from build123d import *

# Parameters (mm, degrees)
SKETCH1_W                                       = 22
SKETCH1_H                                       = 22
BOSS_EXTRUDE1_DEPTH                             = 10
F_1_4_CLEARANCE_HOLE1_D                         = 6.7564
SKETCH6_R                                       = 4
CUT_EXTRUDE1_DEPTH                              = 207.717198123
SKETCH7_R                                       = 12
CUT_EXTRUDE2_DEPTH                              = 207.717198123
CBORE_FOR_10_SOCKET_HEAD_CAP_SCREW1_D           = 5.6134
CBORE_FOR_10_SOCKET_HEAD_CAP_SCREW1_CBORE_D     = 9.525
CBORE_FOR_10_SOCKET_HEAD_CAP_SCREW1_CBORE_DEPTH = 4.826
BOSS_EXTRUDE2_DEPTH                             = 10
BOSS_EXTRUDE2_DEPTH_BACK                        = 10
CBORE_FOR_M3_SHCS1_D                            = 3.6
CBORE_FOR_M3_SHCS1_CBORE_D                      = 6.5
CBORE_FOR_M3_SHCS1_CBORE_DEPTH                  = 3
FILLET1_R                                       = 3
FILLET2_R                                       = 3
FILLET3_R                                       = 10
FILLET4_R                                       = 2


with BuildPart() as part:
    # Sketch1 → Boss-Extrude1 (new body)
    with BuildSketch(Plane(origin=(0, 0, 0), x_dir=(1, 0, 0), z_dir=(0, 1, 0))):
        with Locations((15, 15)):
            Rectangle(SKETCH1_W, SKETCH1_H)
        Polygon((50, 50), (50, 58.485281374), (17.514718626, 26), (26, 26), (26, 17.514718626), (58.485281374, 50), align=None)
        Polygon((50, 75), (50, 100), (75, 100), (100, 100), (100, 50), (75, 50), (50, 50), align=None)
        Polygon((100, 50), (91.514718626, 50), (124, 17.514718626), (124, 26), (132.485281374, 26), (100, 58.485281374), align=None)
        with Locations((135, 15)):
            Rectangle(SKETCH1_W, SKETCH1_H)
        with Locations((135, 135)):
            Rectangle(SKETCH1_W, SKETCH1_H)
        Polygon((124, 132.485281374), (91.514718626, 100), (100, 100), (100, 91.514718626), (132.485281374, 124), (124, 124), align=None)
        Polygon((17.514718626, 124), (50, 91.514718626), (50, 100), (58.485281374, 100), (26, 132.485281374), (26, 124), align=None)
        with Locations((15, 135)):
            Rectangle(SKETCH1_W, SKETCH1_H)
    extrude(amount=-BOSS_EXTRUDE1_DEPTH)

    # 1/4 Clearance Hole1 (through all)
    with Locations(Plane(origin=(0, 0, 0), x_dir=(1, 0, 0), z_dir=(0, 1, 0))):
        with Locations((15, 15), (15, 135), (135, 135), (135, 15)):
            Hole(F_1_4_CLEARANCE_HOLE1_D / 2)

    # Sketch6 → Cut-Extrude1 (cut, through all)
    with BuildSketch(Plane.XZ.offset(10)):
        with Locations(Location((75, -75, 0), (0, 0, 270))):
            Circle(SKETCH6_R)
    extrude(amount=-CUT_EXTRUDE1_DEPTH, mode=Mode.SUBTRACT)

    # Sketch7 → Cut-Extrude2 (cut, through all)
    with BuildSketch(Plane(origin=(0, -10, 0), x_dir=(1, 0, 0), z_dir=(0, 1, 0))):
        with Locations(Location((75, 75, 0), (0, 0, 270))):
            Circle(SKETCH7_R)
    extrude(amount=CUT_EXTRUDE2_DEPTH, mode=Mode.SUBTRACT)

    # CBORE for #10 Socket Head Cap Screw1 (through all)
    with Locations(Plane(origin=(0, -10, 0), x_dir=(-1, 0, 0), z_dir=(0, -1, 0))):
        with Locations((-92.45, 75), (-66.275, 59.887856704), (-66.275, 90.112143296)):
            CounterBoreHole(CBORE_FOR_10_SOCKET_HEAD_CAP_SCREW1_D / 2, CBORE_FOR_10_SOCKET_HEAD_CAP_SCREW1_CBORE_D / 2, CBORE_FOR_10_SOCKET_HEAD_CAP_SCREW1_CBORE_DEPTH)

    # Sketch10 → Boss-Extrude2 (add, two sides: drawn at the far end of the back side and taken through both)
    with BuildSketch(Plane.ZY.offset(-75).offset(-BOSS_EXTRUDE2_DEPTH_BACK)):
        Polygon((-100, -10), (-100, 0), (-87.5, 33.704367651), (-78.5, 33.704367651), (-78.5, 38.704367651), (-87.5, 38.704367651), (-94.178104684, 38.704367651), (-108.532463759, 0), (-108.532463759, -10), align=None)
        Polygon((-71.5, 33.704367651), (-71.5, 38.704367651), (-62.5, 38.704367651), (-55.821895316, 38.704367651), (-41.467536241, 0), (-41.467536241, -10), (-50, -10), (-50, 0), (-62.5, 33.704367651), align=None)
    extrude(amount=BOSS_EXTRUDE2_DEPTH + BOSS_EXTRUDE2_DEPTH_BACK)

    # CBORE for M3 SHCS1 (through all)
    with Locations(Plane(origin=(0, 33.704367651, 0), x_dir=(-1, 0, 0), z_dir=(0, -1, 0))):
        with Locations((-75, 83.5), (-75, 66.5)):
            CounterBoreHole(CBORE_FOR_M3_SHCS1_D / 2, CBORE_FOR_M3_SHCS1_CBORE_D / 2, CBORE_FOR_M3_SHCS1_CBORE_DEPTH)

    # Fillet1
    fillet1_edges = [part.edges().sort_by_distance(p)[0] for p in [
        (85, -5, -108.532463759),
        (85, 36.204367651, -78.5),
        (85, -5, -100),
        (65, -5, -100),
        (65, 36.204367651, -78.5),
        (65, -5, -108.532463759),
        (85, -5, -50),
        (85, 36.204367651, -71.5),
        (85, -5, -41.467536241),
        (65, -5, -41.467536241),
        (65, 36.204367651, -71.5),
        (65, -5, -50),
        (100, -5, -58.485281374),
        (132.485281374, -5, -26),
        (146, -5, -26),
        (146, -5, -4),
        (124, -5, -4),
        (124, -5, -17.514718626),
        (91.514718626, -5, -50),
        (58.485281374, -5, -50),
        (26, -5, -17.514718626),
        (26, -5, -4),
        (4, -5, -4),
        (4, -5, -26),
        (17.514718626, -5, -26),
        (50, -5, -58.485281374),
        (50, -5, -91.514718626),
        (17.514718626, -5, -124),
        (4, -5, -124),
        (4, -5, -146),
        (26, -5, -146),
        (26, -5, -132.485281374),
        (58.485281374, -5, -100),
        (91.514718626, -5, -100),
        (124, -5, -132.485281374),
        (124, -5, -146),
        (146, -5, -146),
        (146, -5, -124),
        (132.485281374, -5, -124),
        (100, -5, -91.514718626),
    ]]
    fillet(fillet1_edges, radius=FILLET1_R)

    # Fillet2
    fillet2_edges = [part.edges().sort_by_distance(p)[0] for p in [
        (85, 0, -48.5),
        (85, 0, -101.5),
        (65, 0, -48.5),
        (65, 0, -101.5),
        (75, 0, -50),
        (75, 0, -100),
    ]]
    fillet(fillet2_edges, radius=FILLET2_R)

    # Fillet3
    fillet3_edges = [part.edges().sort_by_distance(p)[0] for p in [
        (75, 38.704367651, -94.178104684),
        (75, 38.704367651, -55.821895316),
    ]]
    fillet(fillet3_edges, radius=FILLET3_R)

    # Fillet4
    # the kernel refuses this fillet: 2 mm, written as the material it takes off along each edge
    with BuildSketch(Plane(origin=(63, 38.704367651, -71.5), x_dir=(0, 0, 1), z_dir=(1, 0, 0)), Plane(origin=(87, 38.704367651, -78.5), x_dir=(0, 0, -1), z_dir=(-1, 0, 0))) as fillet4_piece_1:
        with BuildLine():
            CenterArc((FILLET4_R, FILLET4_R), FILLET4_R, 180, 90)
            Line((0, FILLET4_R), (0, 0))
            Line((0, 0), (FILLET4_R, 0))
        make_face()
    extrude(amount=24, mode=Mode.SUBTRACT)


solid = part.part
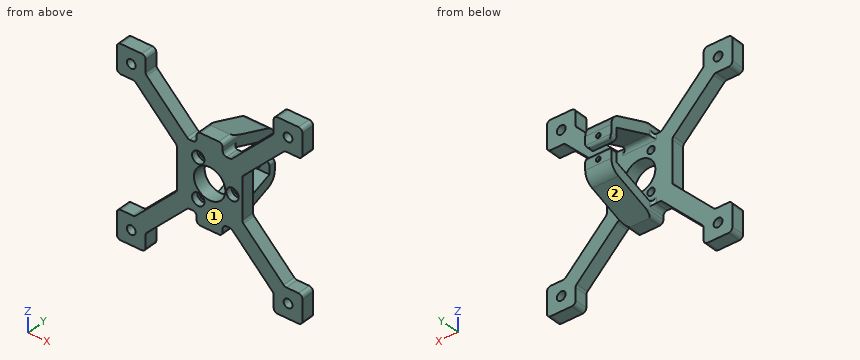
CAD build for the part. Positions are in the model's coordinates, mm. Face numbers are marked on the shaded views. Round coordinates to 2 decimals unless told otherwise and drop trailing zeros. Write each loop counter-clockwise with the first axis right and the second up, starting at its lowest first coordinate (ties: lowest second). Pieces come first, ordered by that corner, then holes.
(1) Mould opens along Y. For the marked faces 1 and 2 say: pulls with the +Y half, pulls with the -Y half, needs draft (parallel to the pull), parting line crosses it, or undercut.
(2) Slice it at C-C, the plane y = 26. Write the cut outline in (x, z).
(3) Drop flat-ended pins along their axis: P1, Ø8, axis at y = 33.5, z = -71.5, coming from the +X side; P2, Ø5, axis at y = -3, z = -72, coming from the -X side; P3, Ø5.5, axis at x = 15, z = -15, coming from the -Y side; P4, Ø6, axis at x = 75, z = -66.5, coming from the +Y side. Give the stop position or say it passes through.
(4) Probe line 1 along Z through (x, y) = (15, -3.75); line 2 along X through (y, z) = (-7, -75); line 3 along X through (y, z) = (38.1, -66.5). List the from-to ranges inside material, lowest first.
(5) Slice it at A-A, the plane z = -75. Write the cut outline in (x, y), and give its area (3 significant figures).
(6) Slice it at D-D, the plane z = -36. Write the cut outline in (x, y).
(7) Slice it at B-B, the plane x = 75. Count the separate pieces of the cut face and the enclosed holes in it, and give its area (3 significant figures).
From the geometry:
1. face 1: pulls with the -Y half
1. face 2: pulls with the +Y half
2. outline: (65, -98.89) - (85, -98.89) - (85, -90.36) - (65, -90.36) - close; (65, -59.64) - (85, -59.64) - (85, -51.11) - (65, -51.11) - close
3. P1: stops at x = 85
3. P2: stops at x = 50
3. P3: passes through
3. P4: stops at y = 38.7
4. line 1: z = -146 to -138.38, -131.62 to -124, -26 to -18.38, -11.62 to -4
4. line 2: x = 50 to 63, 87 to 87.69, 97.21 to 100
4. line 3: x = 65 to 73.2, 76.8 to 85
5. outline: (50, -10) - (63, -10) - (63, 0) - (50, 0) - close; (87, -10) - (87.69, -10) - (87.69, -5.17) - (89.64, -5.17) - (89.64, 0) - (87, 0) - close; (95.26, -5.17) - (97.21, -5.17) - (97.21, -10) - (100, -10) - (100, 0) - (95.26, 0) - close
5. area: 185 mm2
6. outline: (27.51, -10) - (44.49, -10) - (44.49, 0) - (27.51, 0) - close; (105.51, -10) - (122.49, -10) - (122.49, 0) - (105.51, 0) - close
7. separate pieces: 4
7. enclosed holes: 0
7. area: 1,110 mm2
